Verification items for the finished model (mm, model axes). Face numbers are marked on the shaded views. Give positions to 0.01 mm unless a question says otherwise; leave off trailing zeros. Loops run counter-clockwise (first coordinate to the right, second up) from the corner with the lowest first, then second, coordinate; pieces in that order, holes last. Notation, with made-up numbers: (54, 49.25) - (112, 49.25) arc R25 ccw to (112, 74.25) - close; hole circle Ø8 at (60, 31.25). An arc over 180 degrees is marked (long way). One line per question, with ' | ' between items. Start each with the question number.
1. Mould release check, pull along Z, two halves, no side actions. Record for the marked faces 1 and 2: +Z half, -Z half, draft (parallel to the pull), parting line (faces both ways), or undercut.
2. Section check D-D, the plane z = 1.15. State how many separate pieces and enclosed holes the cut face has, then the cut area to 3 significant figures.
3. Section check C-C, the plane x = 62. Enter the section's corners in (y, z) (3 decimals), then the cut area to 3 significant figures.
4. Section check A-A, the plane x = 0. Enter the section's corners in (y, z) (1 decimal), then the cut area to 3 significant figures.
5. Thickness scan on line 1 along X through (y, z) = (60, 2.9); line 2 along Y through (x, z) = (58.5, 0.7); line 3 along X through (y, z) = (32, 2.2). Record the ranges inside material, lowest first. Write a range as from..to.
from build123d import *

# Parameters (mm, degrees)
F0_W     = 152.4
F0_H     = 152.4
F0_R     = 65.0875
F1_DEPTH = 3.175
F3_D     = 6.35


with BuildPart() as f1:
    # F0 (on Top) → F1 (new body)
    with BuildSketch(Plane.XY):
        Rectangle(F0_W, F0_H)
        Circle(F0_R, mode=Mode.SUBTRACT)
    extrude(amount=F1_DEPTH)

    # F3 (through all)
    with Locations(Plane.XY.offset(3.175)):
        with Locations((-61.11317, -61.11317), (61.11317, -61.11317), (61.11317, 61.11317), (-61.11317, 61.11317)):
            Hole(F3_D / 2)


solid = f1.part
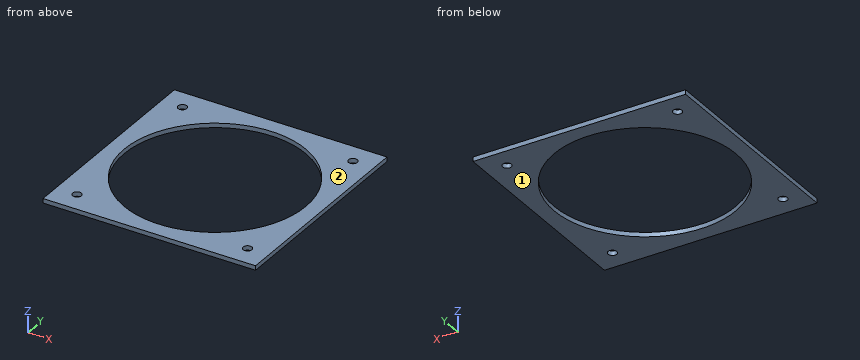
Results list:
1) face 1: -Z half | face 2: +Z half
2) separate pieces: 1 | enclosed holes: 5 | area: 9,790 mm²
3) outline: (-76.2, 0) - (-64.162, 0) - (-64.162, 3.175) - (-76.2, 3.175) - close; (-58.065, 0) - (-19.809, 0) - (-19.809, 3.175) - (-58.065, 3.175) - close; (19.809, 0) - (58.065, 0) - (58.065, 3.175) - (19.809, 3.175) - close; (64.162, 0) - (76.2, 0) - (76.2, 3.175) - (64.162, 3.175) - close | area: 319 mm²
4) outline: (-76.2, 0) - (-65.1, 0) - (-65.1, 3.2) - (-76.2, 3.2) - close; (65.1, 0) - (76.2, 0) - (76.2, 3.2) - (65.1, 3.2) - close | area: 70.6 mm²
5) line 1: -76.2..-64.09, -58.14..-25.23, 25.23..58.14, 64.09..76.2 | line 2: -76.2..-62.92, -59.31..-28.53, 28.53..59.31, 62.92..76.2 | line 3: -76.2..-56.68, 56.68..76.2
